Build history of the part. All positions in model axes, mm. A direction names the side the tool comes from. Coordinates: 2 decimals unless noted, no trailing zeros. Order: outer loops, then holes, each group sorted by start corner. A loop starts at its lowest first (then second) coordinate and runs counter-clockwise, first axis right, second up. Notation, with made-up numbers: (44.5, 87) - (58.5, 87) arc R10 ccw to (58.5, 105) - close; hole circle Ø6 at (68, 50.5). An arc over 180 degrees is marked (long way). One line per item, written item: value.
from build123d import *

# Parameters (mm, degrees)
F0_W     = 3.556
F0_H     = 3.556
F0_W_2   = 15.24
F1_DEPTH = 114.3


with BuildPart() as f1:
    # F0 (on Top) → F1 (new body)
    with BuildSketch(Plane.XY):
        Polygon((-7.62, -3.175), (-7.62, 3.175), (-7.62, 6.731), (-11.176, 6.731), (-11.176, -6.731), (-7.62, -6.731), align=None)
        with Locations((-9.398, 8.509)):
            Rectangle(F0_W, F0_H)
        with Locations((-9.398, -8.509)):
            Rectangle(F0_W, F0_H)
        with Locations((0, -4.953)):
            Rectangle(F0_W_2, F0_H)
        with Locations((0, 4.953)):
            Rectangle(F0_W_2, F0_H)
    extrude(amount=F1_DEPTH)


solid = f1.part
1. 3-axis set-ups, long thin cutter, end or side, ignore diameter. For faces 1 (the face through (0, -6.731, 56)), 2 (the face through (0, -3.175, 56)), 3 (the face through (0, 6.731, 56)), 4 (the face through (-4, -4, 0)): which of +Z, -Z, +X, -X, +Y, -Y reach the whole face in a straight line?
Values found:
face 1: +Z, -Z, +X, -Y
face 2: +Z, -Z, +X
face 3: +Z, -Z, +X, +Y
face 4: -Z, +X, -X, +Y, -Y
2. Band-saw the part on A-A, the plane x = -5. Give the cut face in (y, z) (3 decimals), and give its area (3 significant figures).
Values found:
outline: (-6.731, 0) - (-3.175, 0) - (-3.175, 114.3) - (-6.731, 114.3) - close; (3.175, 0) - (6.731, 0) - (6.731, 114.3) - (3.175, 114.3) - close
area: 813 mm2
3. Band-saw the part on C-C, the plane y = -0.5. Give the cut face in (x, z), and give its area (3 significant figures).
Values found:
outline: (-11.18, 0) - (-7.62, 0) - (-7.62, 114.3) - (-11.18, 114.3) - close
area: 406 mm2
4. Band-saw the part on B-B, the plane z = 28. Give the cut face in (x, y) (3 decimals).
Values found:
outline: (-11.176, -10.287) - (-7.62, -10.287) - (-7.62, -6.731) - (7.62, -6.731) - (7.62, -3.175) - (-7.62, -3.175) - (-7.62, 3.175) - (7.62, 3.175) - (7.62, 6.731) - (-7.62, 6.731) - (-7.62, 10.287) - (-11.176, 10.287) - close
5. Probe line 1 along Y through (x, z) = (2.75, 23) (3 decimals); line 2 along X through (y, z) = (1.5, 51.5). List the from-to ranges inside material, lowest first.
Values found:
line 1: y = -6.731 to -3.175, 3.175 to 6.731
line 2: x = -11.18 to -7.62
6. Flat gauge pins, fed straight in: P1, Ø1, axis at x = -6.5, z = 77, coming from the +Y side; P2, Ø1, axis at y = 0, z = 59, coming from the +X side. Where does each tip first touch, or does it go through?
Values found:
P1: stops at y = 6.73
P2: stops at x = -7.62
